The listing builds one solid part. Answer for the finished solid, in the listing's coordinates (mm). A direction names the side the tool comes from. Round coordinates to 2 decimals unless told otherwise and drop trailing zeros. Write each loop counter-clockwise with the first axis right and the second up, starting at its lowest first coordinate (ties: lowest second). Pieces come first, ordered by that corner, then holes.
Autodesk Inventor part; units mm, degrees
ref_plane "РабПлоскость1" through (0, 13, 0) normal (0, 1, 0) x (1, 0, 0)
ref_plane "YZ Plane" through (0, 0, 0) normal (1, 0, 0) x (0, 1, 0)
ref_plane "XZ Plane" through (0, 0, 0) normal (0, 1, 0) x (-1, 0, 0)
sketch "Эскиз1" plane through (0, 0, 0) normal (0, 1, 0) x (-1, 0, 0)
  line L0 (3, -3) -> (-3, -3)
  line L1 (-3, -3) -> (-3, 3)
  line L2 (-3, 3) -> (3, 3)
  line L3 (3, 3) -> (3, -3)
  line L4 (4.2, 0) -> (-4.2, 0)
  line L5 (0, -4.2) -> (0, 4.2)
  point P0 (0, 0)
  dimension "d0" = 6
  dimension "d1" = 6
extrude "Выдавливание1" add sketch "Эскиз1" along normal blind 4
sketch "Эскиз2" plane through (0, 4, 0) normal (0, 1, 0) x (1, 0, 0)
  circle A0 centre (0, 0) radius 1.5
  dimension "d4" = 3
ref_plane "РабПлоскость1" through (0, 13, 0) normal (0, 1, 0) x (1, 0, 0)
sketch "Эскиз3" plane through (0, 13, 0) normal (0, 1, 0) x (1, 0, 0)
  circle A0 centre (0, 0) radius 1.5
  dimension "d6" = 3
loft "Лофт1" add profiles "Эскиз3", "Эскиз2"
sketch "Эскиз4" plane through (0, 0, 0) normal (0, 0, 1) x (1, 0, 0)
  line L0 (3, 0) -> (-3, 0)
  line L1 (3, 0) -> (3, 4)
  line L2 (-3, 4) -> (3, 4)
  line L3 (-3, 0) -> (-3, 4)
  arc A0 (3.25, 0.5) -> (3, 0.75) centre (3, 0.5) ccw
  line L4 (3.25, 0.5) -> (3.25, -2)
  line L5 (0, -5) -> (0, 16)
  arc A1 (-3, 0.75) -> (-3.25, 0.5) centre (-3, 0.5) ccw
  line L6 (-3.25, 0.5) -> (-3.25, -2)
  point P0 (0, 0)
  dimension "d11" = 0.5
  dimension "d12" = 0.5
  dimension "d13" = 2
sketch "Эскиз5" plane through (3, 0, 3) normal (1, 0, 0) x (0, 0, -1)
  line L0 (3.7546, 0.75) -> (2.4212, 0.75)
  line L1 (0.5, 0.85) -> (1, 0.85)
  line L2 (1, 0.85) -> (1, 0.65)
  line L3 (1, 0.65) -> (0.5, 0.65)
  line L4 (0.5, 0.65) -> (0.5, 0.85)
  line L5 (3, -5) -> (3, 16)
  line L6 (5.5, 0.85) -> (5, 0.85)
  line L7 (5, 0.85) -> (5, 0.65)
  line L8 (5, 0.65) -> (5.5, 0.65)
  line L9 (5.5, 0.65) -> (5.5, 0.85)
  line L10 (3, 0.75) -> (3, 0.5)
  point P0 (3, 0)
  dimension "d14" = 0.5
  dimension "d15" = 0.2
  dimension "d16" = 2
sketch "Эскиз6" plane through (-3, 0, -3) normal (-1, 0, 0) x (0, 0, 1)
  line L0 (5.5, 0.85) -> (5, 0.85)
  line L1 (5.5, 0.65) -> (5.5, 0.85)
  line L2 (5, 0.65) -> (5.5, 0.65)
  line L3 (5, 0.85) -> (5, 0.65)
  line L4 (0, 0) -> (6, 0)
  line L5 (0, 0) -> (0, 4)
  line L6 (6, 4) -> (0, 4)
  line L7 (6, 0) -> (6, 4)
  line L8 (0.5, 0.85) -> (1, 0.85)
  line L9 (1, 0.85) -> (1, 0.65)
  line L10 (1, 0.65) -> (0.5, 0.65)
  line L11 (0.5, 0.65) -> (0.5, 0.85)
  point P0 (3, 0)
sweep "Сдвиг1" add profiles "Эскиз5" path "Эскиз4" path curves A0 L4
sweep "Сдвиг2" add profiles "Эскиз6" path "Эскиз4" path curves A1 L6 contours L1 L2 L3 L0 | L8 L9 L10 L11
sketch "Эскиз7" plane through (0, 0, 0) normal (0, -1, 0) x (1, 0, 0)
  line L0 (-3.35, -2) -> (-3.35, -2.5)
  line L1 (-3.35, -2.5) -> (-3.15, -2.5)
  line L2 (-3.15, -2.5) -> (-3.15, -2)
  line L3 (-3.15, -2) -> (-3.35, -2)
  circle A0 centre (-3.25, -2.25) radius 0.2693
  point P0 (0, 0)
equation "\"d1\" = d0"
properties part number "button"
1. Section C-C on y = 7.5 is taken. Determine the outline of the cut face in (x, z).
Geometry says:
outline: circle Ø3 at (0, 0)
2. Section D-D on z = 1 is taken. Determine the outline of the cut face in (x, y).
Geometry says:
outline: (-3, 0) - (3, 0) - (3, 4) - (1.12, 4) - (1.12, 13) - (-1.12, 13) - (-1.12, 4) - (-3, 4) - close
3. Section A-A on z = 2.35 is taken. Determine the outline of the cut face in (x, y), plus the area to 3 significant figures.
Geometry says:
outline: (-3.35, -2) - (-3.15, -2) - (-3.15, 0.5) arc R0.15 cw to (-3, 0.65) - (-3, 0) - (3, 0) - (3, 0.65) arc R0.15 cw to (3.15, 0.5) - (3.15, -2) - (3.35, -2) - (3.35, 0.5) arc R0.35 ccw to (3, 0.85) - (3, 4) - (-3, 4) - (-3, 0.85) arc R0.35 ccw to (-3.35, 0.5) - close
area: 25.2 mm2
4. Given pin 1 (3 mm diameter, centred on y = 3, z = 1, fed in from +X); pin 2 (1 mm diameter, centred on x = 2.5, z = -1.5, fed in from +Y); pin 3 (2 mm diameter, centred on y = 6.5, z = -0.5, fed in from +X), each flat-ended and moving along its own axis, determine where each tip first touches the part or whether it passes through.
Geometry says:
pin 1: stops at x = 3
pin 2: stops at y = 4
pin 3: stops at x = 1.5
5. Straight lines are drawn through the part: line 1 along X through (y, z) = (-0.5, -2.2); line 2 along X through (y, z) = (1.25, 0.55); line 3 along Y through (x, z) = (-0.25, 0.3). For each, find the intervals that lie inside material, in ascending order.
Geometry says:
line 1: x = -3.35 to -3.15, 3.15 to 3.35
line 2: x = -3 to 3
line 3: y = 0 to 13
6. Section B-B on x = 0 is taken. Determine the outline of the cut face in (y, z), plus the area to 3 significant figures.
Geometry says:
outline: (0, -3) - (4, -3) - (4, -1.5) - (13, -1.5) - (13, 1.5) - (4, 1.5) - (4, 3) - (0, 3) - close
area: 51.0 mm2
7. A tool of negligible diameter and unlimited length cuts with its end or side. For faces 1 (the face through (1.4, 4, 1.4)), 2 (the face through (0, 2, 3)), from which of +Z, -Z, +X, -X, +Y, -Y can it reach the whole face along a straight path? Write none if from no direction.
Geometry says:
face 1: +Y
face 2: +Z, +X, -X, +Y, -Y
